The figure shows three views and two pictorial views of one solid part (mm, origin at its lowest corner). Answer the questions. Round coordinates to 2 decimals unless told otherwise and drop trailing zeros. Loops run counter-clockwise (first coordinate to the right, second up) from the corner with the lowest first, then second, coordinate; pieces in that order, holes last. Notation, with made-up numbers: (41.5, 44.5) -> (57.5, 44.5) arc R30 ccw to (57.5, 81.5) -> close; hole circle Ø8 at (-36.75, -19.75). An arc over 180 degrees is marked (long way). Write each question's results on one line, items separated by ' | '. Start each with the question number.
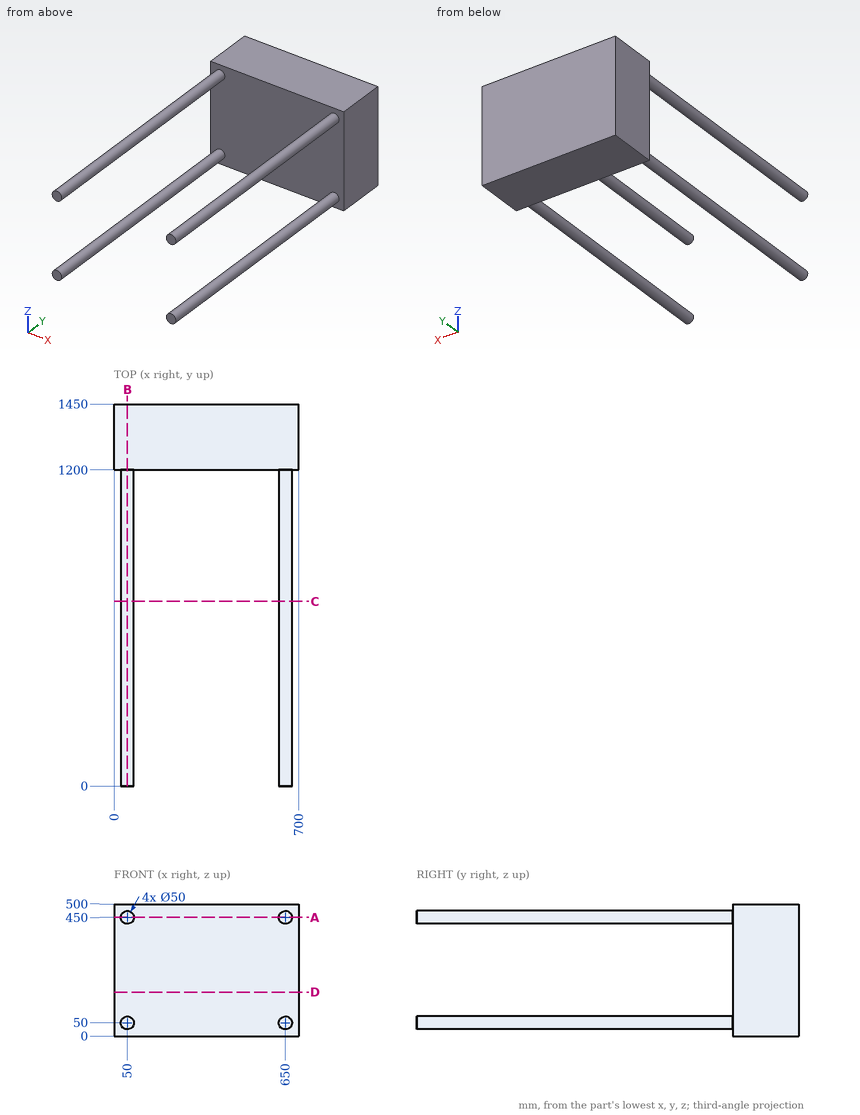
Item 1: The part is cut by section C-C, the plane y = 701. Give the vertices of the cut face in (x, z), plus the area to 3 significant figures.
Item 2: Each of these flat-tipped pins is pushed along its axis until it touches: pin 1 Ø8 at (x, y) = (626.5, 884) entering from +Z; pin 2 Ø10 at (x, z) = (258.5, 107.5) entering from -Y. Where does it stop, or does it pass through?
Item 3: Straight lines are drawn through the part: L1, parallel to X at y = 1171, z = 52.5; L2, parallel to Y at x = 581, z = 315.5; L3, parallel to X at y = 86, z = 460. For each, find the intervals that lie inside material, in ascending order. Write a range as [from, to].
Item 4: The part is cut by section B-B, the plane x = 50. Give the vertices of the cut face in (y, z), plus the area to 3 significant figures.
Item 5: The part is cut by section D-D, the plane z = 166. Give the vertices of the cut face in (x, y).
Item 6: The part is cut by section A-A, the plane z = 450. Give the vertices of the cut face in (x, y), plus the area to 3 significant figures.
Report:
1) outline: circle Ø50 at (50, 50); circle Ø50 at (50, 450); circle Ø50 at (650, 50); circle Ø50 at (650, 450) | area: 7,850 mm2
2) pin 1: stops at z = 465.64 | pin 2: stops at y = 1200
3) L1: x = [25.13, 74.87], [625.13, 674.87] | L2: y = [1200, 1450] | L3: x = [27.09, 72.91], [627.09, 672.91]
4) outline: (0, 25) -> (1200, 25) -> (1200, 0) -> (1450, 0) -> (1450, 500) -> (1200, 500) -> (1200, 475) -> (0, 475) -> (0, 425) -> (1200, 425) -> (1200, 75) -> (0, 75) -> close | area: 245,000 mm2
5) outline: (0, 1200) -> (700, 1200) -> (700, 1450) -> (0, 1450) -> close
6) outline: (0, 1200) -> (25, 1200) -> (25, 0) -> (75, 0) -> (75, 1200) -> (625, 1200) -> (625, 0) -> (675, 0) -> (675, 1200) -> (700, 1200) -> (700, 1450) -> (0, 1450) -> close | area: 295,000 mm2
